The model under review builds one solid part; all positions refer to its coordinate system, in mm. Face numbers are marked on the shaded views. A direction names the side the tool comes from. Round coordinates to 2 decimals unless told otherwise and drop trailing zeros. Order: outer loops, then holes, each group sorted by start corner. A loop starts at its lowest first (then second) coordinate and runs counter-clockwise, first axis right, second up. Notation, with made-up numbers: M -16.5,-23.5 L 27.5,-23.5 A7 ccw 27.5,-12.5 Z; hole C -21,43.25 d1. An arc over 180 degrees is marked long. Use a Markdown table: item, result. Add a question column.
1. To check wall thickness, follow probe 1 along Y at (x, z) = (-35.5, 0.5); probe 2 along X at (y, z) = (-29, 6); probe 3 along X at (y, z) = (-12.5, 3). State the ranges of each line that lie inside material, in increasing order.
2. Consider section D-D on y = -29.5. Count the separate pieces of the cut face and the enclosed holes in it, then the cut area to 3 significant figures.
3. For the marked faces 1, 2 and 3, list the 3-axis set-ups (+Z, -Z, +X, -X, +Y, -Y) from which the entire face can be reached by the end or side of a thin tool; tool diameter is ignored.
4. Insertion check: P1, Ø5, axis at x = 34.37, y = -11.75, coming from the -Z side; P2, Ø3, axis at x = 27, y = -9.5, coming from the -Z side (3 decimals); P3, Ø7, axis at x = -34.53, y = -27.75, coming from the -Z side; P4, Ø19.5, axis at x = -13, y = -17, coming from the -Z side. Each pin has a flat end and moves straight along its axis. Give the tip position at first contact, or say it passes through.
5. Consider section C-C on z = -16. State the section outline as (x, y) points.
6. The part is to be moulded in two halves that separate along X. For the marked faces 4, 5, 6 and 7, say which applies: +X half, -X half, draft (parallel to the pull), parting line (faces both ways), or undercut.
7. Consider section A-A on y = -11.75. State the section outline as (x, z) points.
8. Consider section B-B on y = -24. State the section outline as (x, z) points.
from build123d import *

# Parameters (mm, degrees)
SKETCH4_W           = 78.9
SKETCH4_H           = 39.3
BOSS_EXTRUDE2_DEPTH = 8
CUT_EXTRUDE2_REACH  = 58.315
CUT_EXTRUDE3_REACH  = 58.315
SKETCH7_R           = 2.65
CHAMFER3_SIZE       = 1
CHAMFER4_SIZE       = 0.5
SKETCH8_W           = 54.974490404
SKETCH8_H           = 5
BOSS_EXTRUDE3_DEPTH = 24.4
FILLET1_R           = 8


with BuildPart() as part:
    # Sketch4 → Boss-Extrude2 (new body)
    with BuildSketch(Plane.XY):
        with Locations((-0.082754798, -19.65)):
            Rectangle(SKETCH4_W, SKETCH4_H)
    extrude(amount=BOSS_EXTRUDE2_DEPTH)

    # Sketch6 → Cut-Extrude2 (cut, up to next)
    with BuildSketch(Plane.XY.offset(8), mode=Mode.PRIVATE) as cut_extrude2_sk1:
        with BuildLine():
            Line((28.287245202, -39.5), (28.287245202, -34.966633333))
            ThreePointArc((28.287245202, -34.966633333), (24.090185885, -28.57821772), (17.597136747, -32.611513376))
            ThreePointArc((17.597136747, -32.611513376), (17.234869858, -32.976161871), (16.742475109, -32.828672095))
            ThreePointArc((16.742475109, -32.828672095), (13.426365224, -31.57225608), (10.450959192, -33.501537013))
            ThreePointArc((10.450959192, -33.501537013), (10.018755802, -33.750140454), (9.586552412, -33.501537013))
            ThreePointArc((9.586552412, -33.501537013), (5.626846324, -31.591156717), (2.378419018, -34.553680172))
            ThreePointArc((2.378419018, -34.553680172), (2.064006845, -34.905939189), (1.596551631, -34.839403086))
            ThreePointArc((1.596551631, -34.839403086), (0.102573651, -34.35), (-1.39140433, -34.839403086))
            ThreePointArc((-1.39140433, -34.839403086), (-1.858859544, -34.905939189), (-2.173271717, -34.553680172))
            ThreePointArc((-2.173271717, -34.553680172), (-5.421699023, -31.591156717), (-9.381405111, -33.501537013))
            ThreePointArc((-9.381405111, -33.501537013), (-9.813608501, -33.750140454), (-10.245811891, -33.501537013))
            ThreePointArc((-10.245811891, -33.501537013), (-13.71465449, -31.550736756), (-17.105314368, -33.634463277))
            ThreePointArc((-17.105314368, -33.634463277), (-17.289281672, -33.828504165), (-17.54693295, -33.9))
            Line((-17.54693295, -33.9), (-25.852754798, -33.9))
            ThreePointArc((-25.852754798, -33.9), (-27.422811269, -34.381612052), (-28.452754798, -35.660769515))
            Line((-28.452754798, -35.660769515), (-28.452754798, -39.5))
            Line((-28.452754798, -39.5), (28.287245202, -39.5))
        make_face()
    cut_extrude2_tool1 = extrude(cut_extrude2_sk1.sketch, amount=-CUT_EXTRUDE2_REACH, mode=Mode.PRIVATE) & part.part
    add(cut_extrude2_tool1.solids().sort_by_distance((2.671043, -35.689379, 8))[0], mode=Mode.SUBTRACT)

    # Sketch7 → Cut-Extrude3 (cut, up to next)
    with BuildSketch(Plane.XY.offset(8), mode=Mode.PRIVATE) as cut_extrude3_sk1:
        with Locations((-34.532754798, -11.75)):
            Circle(SKETCH7_R)
    cut_extrude3_tool1 = extrude(cut_extrude3_sk1.sketch, amount=-CUT_EXTRUDE3_REACH, mode=Mode.PRIVATE) & part.part
    # Sketch7 → Cut-Extrude3 (cut, up to next)
    with BuildSketch(Plane.XY.offset(8), mode=Mode.PRIVATE) as cut_extrude3_sk2:
        with Locations((-34.532754798, -27.75)):
            Circle(SKETCH7_R)
    cut_extrude3_tool2 = extrude(cut_extrude3_sk2.sketch, amount=-CUT_EXTRUDE3_REACH, mode=Mode.PRIVATE) & part.part
    # Sketch7 → Cut-Extrude3 (cut, up to next)
    with BuildSketch(Plane.XY.offset(8), mode=Mode.PRIVATE) as cut_extrude3_sk3:
        with Locations((34.367245202, -11.75)):
            Circle(SKETCH7_R)
    cut_extrude3_tool3 = extrude(cut_extrude3_sk3.sketch, amount=-CUT_EXTRUDE3_REACH, mode=Mode.PRIVATE) & part.part
    # Sketch7 → Cut-Extrude3 (cut, up to next)
    with BuildSketch(Plane.XY.offset(8), mode=Mode.PRIVATE) as cut_extrude3_sk4:
        with Locations((34.367245202, -27.75)):
            Circle(SKETCH7_R)
    cut_extrude3_tool4 = extrude(cut_extrude3_sk4.sketch, amount=-CUT_EXTRUDE3_REACH, mode=Mode.PRIVATE) & part.part
    add(cut_extrude3_tool1.solids().sort_by_distance((-34.532755, -11.75, 8))[0], mode=Mode.SUBTRACT)
    add(cut_extrude3_tool2.solids().sort_by_distance((-34.532755, -27.75, 8))[0], mode=Mode.SUBTRACT)
    add(cut_extrude3_tool3.solids().sort_by_distance((34.367245, -11.75, 8))[0], mode=Mode.SUBTRACT)
    add(cut_extrude3_tool4.solids().sort_by_distance((34.367245, -27.75, 8))[0], mode=Mode.SUBTRACT)

    # Chamfer3
    chamfer3_edges = [part.edges().sort_by_distance(p)[0] for p in [
        (-0.082754798, 0, 8),
        (-39.532754798, -19.65, 8),
        (33.827245202, -39.3, 8),
        (-28.452754798, -39.3, 4),
        (28.287245202, -39.3, 4),
        (-33.992754798, -39.3, 8),
        (39.367245202, -19.65, 8),
        (-39.532754798, -39.3, 4),
        (-39.532754798, 0, 4),
        (39.367245202, 0, 4),
        (39.367245202, -39.3, 4),
    ]]
    chamfer(chamfer3_edges, length=CHAMFER3_SIZE)

    # Chamfer4
    chamfer4_edges = [part.edges().sort_by_distance(p)[0] for p in [
        (-27.422811269, -34.381612052, 0),
        (-21.699843874, -33.9, 0),
        (-17.289281672, -33.828504165, 0),
        (-13.71465449, -31.550736756, 0),
        (-9.813608501, -33.750140454, 0),
        (-5.421699023, -31.591156717, 0),
        (-1.858859544, -34.905939189, 0),
        (0.102573651, -34.35, 0),
        (2.064006845, -34.905939189, 0),
        (24.090185885, -28.57821772, 0),
        (5.626846324, -31.591156717, 0),
        (17.234869858, -32.976161871, 0),
        (10.018755802, -33.750140454, 0),
        (13.426365224, -31.57225608, 0),
    ]]
    chamfer(chamfer4_edges, length=CHAMFER4_SIZE - 0.0001)  # a hair under: the kernel refuses the full size
    chamfer4_2_edges = [part.edges().sort_by_distance(p)[0] for p in [
        (28.287245202, -37.41718435, 0),
    ]]
    chamfer(chamfer4_2_edges, length=CHAMFER4_SIZE)
    chamfer4_3_edges = [part.edges().sort_by_distance(p)[0] for p in [
        (-27.422811269, -34.381612052, 8),
        (-21.699843874, -33.9, 8),
        (-17.289281672, -33.828504165, 8),
        (-13.71465449, -31.550736756, 8),
        (-9.813608501, -33.750140454, 8),
        (-5.421699023, -31.591156717, 8),
        (-1.858859544, -34.905939189, 8),
        (0.102573651, -34.35, 8),
        (2.064006845, -34.905939189, 8),
        (24.090185885, -28.57821772, 8),
        (5.626846324, -31.591156717, 8),
        (17.234869858, -32.976161871, 8),
        (10.018755802, -33.750140454, 8),
        (13.426365224, -31.57225608, 8),
    ]]
    chamfer(chamfer4_3_edges, length=CHAMFER4_SIZE - 0.0001)  # a hair under: the kernel refuses the full size
    chamfer4_4_edges = [part.edges().sort_by_distance(p)[0] for p in [
        (28.287245202, -37.41718435, 8),
    ]]
    chamfer(chamfer4_4_edges, length=CHAMFER4_SIZE)
    chamfer4_5_edges = [part.edges().sort_by_distance(p)[0] for p in [
        (-28.452754798, -36.980384758, 0),
    ]]
    chamfer(chamfer4_5_edges, length=CHAMFER4_SIZE - 0.0001)  # a hair under: the kernel refuses the full size
    chamfer4_6_edges = [part.edges().sort_by_distance(p)[0] for p in [
        (-28.452754798, -36.980384758, 8),
    ]]
    chamfer(chamfer4_6_edges, length=CHAMFER4_SIZE - 0.0001)  # a hair under: the kernel refuses the full size

    # Sketch8 → Boss-Extrude3 (add)
    with BuildSketch(Plane(origin=(0, 0, 0), x_dir=(-1, 0, 0), z_dir=(0, 0, -1))):
        with Locations((0, -2.5)):
            Rectangle(SKETCH8_W, SKETCH8_H)
    extrude(amount=BOSS_EXTRUDE3_DEPTH)

    # Fillet1
    fillet1_edges = [part.edges().sort_by_distance(p)[0] for p in [
        (0, -5, 0),
    ]]
    fillet(fillet1_edges, radius=FILLET1_R)


solid = part.part
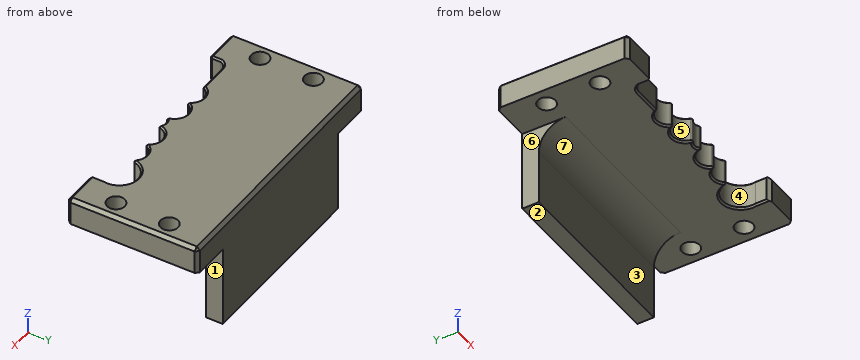
Answer block:
| question | item | result |
|---|---|---|
| 1 | probe 1 | -39.3 to -30.22, -25.28 to -14.22, -9.28 to 0 |
| 1 | probe 2 | -39.53 to -36.87, -32.2 to 20.52, 25.3 to 32.03, 36.7 to 39.37 |
| 1 | probe 3 | -39.53 to -37.07, -31.99 to 31.83, 36.91 to 39.37 |
| 2 | separate pieces | 4 |
| 2 | enclosed holes | 0 |
| 2 | area | 514 mm^2 |
| 3 | face 1 | -Z, +X, +Y, -Y |
| 3 | face 2 | -Z, +X, -X, +Y, -Y |
| 3 | face 3 | -Z, +X, -X, -Y |
| 4 | P1 | through |
| 4 | P2 | z = -1.755 |
| 4 | P3 | z = 0 |
| 4 | P4 | z = -2.44 |
| 5 | outline | M -27.49,-5 L 27.49,-5 L 27.49,0 L -27.49,0 Z |
| 6 | face 4 | undercut |
| 6 | face 5 | undercut |
| 6 | face 6 | -X half |
| 6 | face 7 | draft |
| 7 | outline | M -39.53,0 L -37.18,0 L -37.18,8 L -38.53,8 L -39.53,7 Z; M -31.88,0 L -27.49,0 L -27.49,-0.1 L 27.49,-0.1 L 27.49,0 L 31.72,0 L 31.72,8 L -31.88,8 Z; M 37.02,0 L 39.37,0 L 39.37,7 L 38.37,8 L 37.02,8 Z |
| 8 | outline | M -39.53,0 L 39.37,0 L 39.37,7 L 38.37,8 L -38.53,8 L -39.53,7 Z |
